from build123d import *

# Parameters (mm, degrees)
SZKIC1_W                        = 27
SZKIC1_H                        = 25
ZAOKR_GLENIE1_R                 = 4
SZKIC4_R                        = 3
WYTNIJ_WYCI_GNI_CIE3_DEPTH      = 24.0000001
WYTNIJ_WYCI_GNI_CIE3_DEPTH_BACK = 3
WYTNIJ_WYCI_GNI_CIE2_DEPTH      = 24.0000001
SZKIC5_OUTSIDE_W                = 72.072
SZKIC5_OUTSIDE_H                = 72.072
WYTNIJ_WYCI_GNI_CIE4_DEPTH      = 26.0000001
SZKIC8_W                        = 7.75
SZKIC8_H                        = 13.192742838
SZKIC10_R                       = 3.5
WYTNIJ_WYCI_GNI_CIE5_DEPTH      = 52.807257262


with BuildPart() as part:
    # Szkic1 → Obrót1 (revolve)
    with BuildSketch(Plane.XY):
        with Locations((13.5, 12.5)):
            Rectangle(SZKIC1_W, SZKIC1_H)
    revolve(axis=Axis((0, 0, 0), (0, 1, 0)))

    # Szkic2 → Wycięcie-obrót1 (revolve, cut)
    with BuildSketch(Plane.XY):
        Polygon((27, 25), (27, 2), (7.75, 9.00642701), (7.75, 25), align=None)
    revolve(axis=Axis((0, 0, 0), (0, 1, 0)), mode=Mode.SUBTRACT)

    # Zaokrąglenie1
    zaokr_glenie1_edges = [part.edges().sort_by_distance(p)[0] for p in [
        (-7.75, 9.00642701, 0),
    ]]
    fillet(zaokr_glenie1_edges, radius=ZAOKR_GLENIE1_R)

    # Szkic4 → Wytnij-wyciągnięcie3 (cut, two sides)
    with BuildSketch(Plane(origin=(0, 2, 0), x_dir=(1, 0, 0), z_dir=(0, 1, 0))) as wytnij_wyci_gni_cie3_sk:
        with Locations((-20, 0)):
            Circle(SZKIC4_R)
        with Locations((20, 0)):
            Circle(SZKIC4_R)
    extrude(amount=WYTNIJ_WYCI_GNI_CIE3_DEPTH, mode=Mode.SUBTRACT)
    extrude(wytnij_wyci_gni_cie3_sk.sketch, amount=-WYTNIJ_WYCI_GNI_CIE3_DEPTH_BACK, mode=Mode.SUBTRACT)

    # Szkic3 → Wytnij-wyciągnięcie2 (cut, through all)
    with BuildSketch(Plane(origin=(0, 2, 0), x_dir=(1, 0, 0), z_dir=(0, 1, 0))):
        with BuildLine():
            Line((-17.5, 5), (-26.532998323, 5))
            ThreePointArc((-26.532998323, 5), (-27, 0), (-26.532998323, -5))
            Line((-26.532998323, -5), (-17.5, -5))
            ThreePointArc((-17.5, -5), (-12.5, 0), (-17.5, 5))
        make_face()
        with BuildLine():
            Line((17.5, 5), (26.532998323, 5))
            ThreePointArc((26.532998323, 5), (27, 0), (26.532998323, -5))
            Line((26.532998323, -5), (17.5, -5))
            ThreePointArc((17.5, -5), (12.5, 0), (17.5, 5))
        make_face()
    extrude(amount=WYTNIJ_WYCI_GNI_CIE2_DEPTH, mode=Mode.SUBTRACT)

    # Szkic5 outside → Wytnij-wyciągnięcie4 (cut, through all)
    with BuildSketch(Plane.XZ):
        Rectangle(SZKIC5_OUTSIDE_W, SZKIC5_OUTSIDE_H)
        with BuildLine():
            Line((-20.2625, 6.995076393), (-0.290625, 7.744548864))
            ThreePointArc((-0.290625, 7.744548864), (0, 7.75), (0.290625, 7.744548864))
            Line((0.290625, 7.744548864), (20.2625, 6.995076393))
            ThreePointArc((20.2625, 6.995076393), (27, 0), (20.2625, -6.995076393))
            Line((20.2625, -6.995076393), (0.290625, -7.744548864))
            ThreePointArc((0.290625, -7.744548864), (0, -7.75), (-0.290625, -7.744548864))
            Line((-0.290625, -7.744548864), (-20.2625, -6.995076393))
            ThreePointArc((-20.2625, -6.995076393), (-27, 0), (-20.2625, 6.995076393))
        make_face(mode=Mode.SUBTRACT)
    extrude(amount=-WYTNIJ_WYCI_GNI_CIE4_DEPTH, mode=Mode.SUBTRACT)

    # Szkic8 → Wycięcie-obrót2 (revolve, cut)
    with BuildSketch(Plane.XY):
        with Locations((3.875, 18.403628581)):
            Rectangle(SZKIC8_W, SZKIC8_H)
    revolve(axis=Axis((0, 25, 0), (0, -1, 0)), mode=Mode.SUBTRACT)

    # Szkic9 → Obrót2 (revolve)
    with BuildSketch(Plane.XY):
        Polygon((5.35, 51.807257162), (0, 51.807257162), (0, 11.807257162), (6.3, 11.807257162), (6.3, 48.807257162), (6.35, 48.807257162), (6.35, 50.807257162), align=None)
    revolve(axis=Axis((0, 11.807257162, 0), (0, 1, 0)))

    # Szkic10 → Wytnij-wyciągnięcie5 (cut, through all)
    with BuildSketch(Plane(origin=(0, 51.807257162, 0), x_dir=(1, 0, 0), z_dir=(0, 1, 0))):
        Circle(SZKIC10_R)
    extrude(amount=-WYTNIJ_WYCI_GNI_CIE5_DEPTH, mode=Mode.SUBTRACT)


solid = part.part
Work out the finished part from the listing and answer in its coordinate system (mm). A direction names the side the tool comes from. Round coordinates to 2 decimals unless told otherwise and drop trailing zeros. Write each loop counter-clockwise with the first axis right and the second up, starting at its lowest first coordinate (ties: lowest second). Pieces come first, ordered by that corner, then holes.
1) A cutting plane is placed at A-A (y = 18). Give the vertices of the cut face in (x, z).
2) The mould has two halves that part along Y. Classify faces 1 (the cylindrical face through (-5, 30.57, 3.83)), 2 (the flat face through (-20, 3, -5)), 3 (the flat face through (1.1, 51.807, 3.5)): pulls with the +Y half, pulls with the -Y half, needs draft (parallel to the pull), parting line crosses it, or undercut.
3) Straight lines are drawn through the part: line 1 (X direction, y = 0.65, z = 0); line 2 (X direction, y = 22.5, z = 0); line 3 (Z direction, x = -20, y = 0.6). For each, find the intervals that lie inside material, in ascending order.
4) A tool of negligible diameter and unlimited length cuts with its end or side. For faces 4 (the cylindrical face through (3.233, 26.266, 1.341)), 5 (the flat face through (20, 3, 5)), 6 (the cylindrical face through (-1.38, 49.82, 6.2)), 7 (the flat face through (-23, 2, -1)), from which of +Z, -Z, +X, -X, +Y, -Y can it reach the whole face along a straight path? Write none if from no direction.
5) Given pin 1 Ø5 at (x, z) = (-15, 4) entering from +Y; pin 2 Ø1 at (y, z) = (12, 5) entering from +X; pin 3 Ø3.5 at (x, y) = (22.5, 3) entering from -Z; pin 4 Ø8 at (x, z) = (8, -1.5) entering from +Y, each flat-ended and moving along its own axis, determine where each tip first touches the part or whether it passes through.
6) A cutting plane is placed at B-B (z = 1.25). Give the number of separate pieces and of enclosed holes in the cut face, plus the area to 3 significant figures.
Completed:
1. outline: circle Ø12.6 at (0, 0); hole circle Ø7 at (0, 0)
2. face 1: undercut
2. face 2: needs draft
2. face 3: pulls with the +Y half
3. line 1: x = -27 to -23, -17 to -3.5, 3.5 to 17, 23 to 27
3. line 2: x = -6.3 to -3.5, 3.5 to 6.3
3. line 3: z = -7 to -3, 3 to 7
4. face 4: +Y, -Y
4. face 5: +X, +Y
4. face 6: +Y
4. face 7: -X, +Y
5. pin 1: stops at y = 7.09
5. pin 2: stops at x = 6.28
5. pin 3: stops at z = -6.96
5. pin 4: stops at y = 51.81
6. separate pieces: 4
6. enclosed holes: 0
6. area: 454 mm2
